Here's how the part is built. I have some questions about the finished solid (model axes, mm). A direction names the side the tool comes from. Give positions to 0.01 mm unless a question says otherwise; leave off trailing zeros. Loops run counter-clockwise (first coordinate to the right, second up) from the corner with the lowest first, then second, coordinate; pieces in that order, holes last. Notation, with made-up numbers: (48, -32.5) -> (82, -32.5) arc R32 ccw to (82, -0.5) -> close; hole circle Ø8 at (2.5, 89). An arc over 180 degrees is marked (long way). Answer in a Markdown table with one row per item. Add a question column.
Item 1: If we section it at A-A (z = 93): Give the number of separate pieces and of enclosed holes in the cut face, then the cut area to 3 significant figures.
Item 2: If we section it at B-B (z = 37): Write out the boundary of the cut face in (x, y).
Item 3: If we section it at C-C (y = 85): Write out the boundary of the cut face in (x, z).
Item 4: If we section it at D-D (x = 0): Write out the boundary of the cut face in (y, z).
Item 5: Which directions (+Z, -Z, +X, -X, +Y, -Y) give clear straight access to the entire face, cutting with the end or side of a thin tool? Please do faces 4 (the face through (23.92, 80.12, 75.35)), 5 (the face through (40, -83, 90)), 6 (the face through (-1, 8, 25)).
Item 6: We'd pull the mould along Y, two halves only. Please class faces 1 (the face through (-1, 35, 63)), 2 (the face through (25, 85, 50)), 3 (the face through (-1, -65, 100)): released by +Y, released by -Y, zero draft, split by the parting line, or undercut.
Item 7: For P1, Ø1, axis at y = -28, z = 83.5, coming from the +X side; P2, Ø5, axis at x = -25.5, y = 86, coming from the +Z side, each with a flat end and sliding along its axis, tell me the tip position at first contact or that it passes through.
Item 8: If I drill on line 1 (Y direction, x = -42.5, z = 63); line 2 (Y direction, x = 0, z = 82); line 3 (Z direction, x = -7, y = 14.5), over which ranges is the centre line in solid material (lowest first)?
```python
from build123d import *

# Parameters (mm, degrees)
F0_W     = 100
F0_H     = 135
F1_DEPTH = 100
F0_W_2   = 11.520768702
F0_H_2   = 10
F2_DEPTH = 100
F3_W     = 100
F3_H     = 10
F3_H_2   = 15
F5_DEPTH = 75
F6_DEPTH = 50
F4_W     = 10
F4_H     = 20
F7_DEPTH = 10


with BuildPart() as f1:
    # F0 (on Top) → F1 (new body)
    with BuildSketch(Plane.XY):
        with Locations((0, 32.5)):
            Rectangle(F0_W, F0_H)
    extrude(amount=F1_DEPTH)

    # F0 (on Top) → F2 (join)
    with BuildSketch(Plane.XY):
        Polygon((50, -45), (50, -35), (-50, -35), (-50, -100), (50, -100), (50, -90), (38.479231298, -90), (38.479231298, -80), (50, -80), (50, -55), (38.479231298, -55), (38.479231298, -45), align=None)
        with Locations((44.239615649, -50)):
            Rectangle(F0_W_2, F0_H_2)
        with Locations((44.239615649, -85)):
            Rectangle(F0_W_2, F0_H_2)
    extrude(amount=F2_DEPTH)

    # F3 (on face) → F5 (cut)
    with BuildSketch(Plane.XY.offset(100)):
        with Locations((0, -25)):
            Rectangle(F3_W, F3_H)
        with Locations((0, 7.5)):
            Rectangle(F3_W, F3_H_2)
        with Locations((0, 40)):
            Rectangle(F3_W, F3_H)
    extrude(amount=-F5_DEPTH, mode=Mode.SUBTRACT)

    # F3 (on face) → F6 (cut)
    with BuildSketch(Plane.XY.offset(100)):
        with BuildLine():
            ThreePointArc((20, 65), (25, 60), (30, 65))
            Line((30, 65), (20, 65))
        make_face()
        with BuildLine():
            Line((20, 65), (30, 65))
            ThreePointArc((30, 65), (25, 70), (20, 65))
        make_face()
        with BuildLine():
            ThreePointArc((-5, 65), (0, 60), (5, 65))
            Line((5, 65), (-5, 65))
        make_face()
        with BuildLine():
            Line((-5, 65), (5, 65))
            ThreePointArc((5, 65), (0, 70), (-5, 65))
        make_face()
        with BuildLine():
            Line((-20, 65), (-30, 65))
            ThreePointArc((-30, 65), (-25, 60), (-20, 65))
        make_face()
        with BuildLine():
            ThreePointArc((-20, 65), (-25, 70), (-30, 65))
            Line((-30, 65), (-20, 65))
        make_face()
        with BuildLine():
            ThreePointArc((-30, 85), (-25, 80), (-20, 85))
            Line((-20, 85), (-30, 85))
        make_face()
        with BuildLine():
            Line((-30, 85), (-20, 85))
            ThreePointArc((-20, 85), (-25, 90), (-30, 85))
        make_face()
        with BuildLine():
            Line((-5, 85), (5, 85))
            ThreePointArc((5, 85), (0, 90), (-5, 85))
        make_face()
        with BuildLine():
            ThreePointArc((-5, 85), (0, 80), (5, 85))
            Line((5, 85), (-5, 85))
        make_face()
        with BuildLine():
            ThreePointArc((20, 85), (25, 80), (30, 85))
            Line((30, 85), (20, 85))
        make_face()
        with BuildLine():
            Line((20, 85), (30, 85))
            ThreePointArc((30, 85), (25, 90), (20, 85))
        make_face()
    extrude(amount=-F6_DEPTH, mode=Mode.SUBTRACT)

    # F4 (on face) → F7 (cut)
    with BuildSketch(Plane.YZ.offset(50)):
        with Locations((-82.5, 90)):
            Rectangle(F4_W, F4_H)
        with Locations((-47.5, 90)):
            Rectangle(F4_W, F4_H)
    extrude(amount=-F7_DEPTH, mode=Mode.SUBTRACT)


solid = f1.part
```
Recorded:
| question | item | result |
|---|---|---|
| 1 | separate pieces | 4 |
| 1 | enclosed holes | 6 |
| 1 | area | 15,800 mm^2 |
| 2 | outline | (-50, -100) -> (50, -100) -> (50, -30) -> (-50, -30) -> close; (-50, -20) -> (50, -20) -> (50, 0) -> (-50, 0) -> close; (-50, 15) -> (50, 15) -> (50, 35) -> (-50, 35) -> close; (-50, 45) -> (50, 45) -> (50, 100) -> (-50, 100) -> close |
| 3 | outline | (-50, 0) -> (50, 0) -> (50, 100) -> (30, 100) -> (30, 50) -> (20, 50) -> (20, 100) -> (5, 100) -> (5, 50) -> (-5, 50) -> (-5, 100) -> (-20, 100) -> (-20, 50) -> (-30, 50) -> (-30, 100) -> (-50, 100) -> close |
| 4 | outline | (-100, 0) -> (100, 0) -> (100, 100) -> (90, 100) -> (90, 50) -> (80, 50) -> (80, 100) -> (70, 100) -> (70, 50) -> (60, 50) -> (60, 100) -> (45, 100) -> (45, 25) -> (35, 25) -> (35, 100) -> (15, 100) -> (15, 25) -> (0, 25) -> (0, 100) -> (-20, 100) -> (-20, 25) -> (-30, 25) -> (-30, 100) -> (-100, 100) -> close |
| 5 | face 4 | +Z |
| 5 | face 5 | +Z, +X |
| 5 | face 6 | +Z, +X, -X |
| 6 | face 1 | undercut |
| 6 | face 2 | undercut |
| 6 | face 3 | zero draft |
| 7 | P1 | passes through |
| 7 | P2 | stops at z = 50 |
| 8 | line 1 | y = -100 to -30, -20 to 0, 15 to 35, 45 to 100 |
| 8 | line 2 | y = -100 to -30, -20 to 0, 15 to 35, 45 to 60, 70 to 80, 90 to 100 |
| 8 | line 3 | z = 0 to 25 |
